Read the model definition and answer for the solid it produces. Units are mm, in the model's axes. A direction names the side the tool comes from. Round coordinates to 2 decimals unless told otherwise and drop trailing zeros. Order: outer loops, then holes, each group sorted by start corner. A loop starts at its lowest first (then second) coordinate and runs counter-clockwise, first axis right, second up. Notation, with made-up numbers: (29, 21) -> (84, 21) arc R32 ccw to (84, 56) -> close; hole circle Ø5 at (-32, 8). An arc over 180 degrees is marked (long way). Use a Markdown table: item, result. Add a question column.
1. Given pin 1 (2.5 mm diameter, centred on x = 3.5, y = 21, fed in from -Z); pin 2 (3 mm diameter, centred on x = -17.5, z = 10.5, fed in from +Y); pin 3 (4 mm diameter, centred on y = 14.5, z = 18.5, fed in from +X), each flat-ended and moving along its own axis, determine where each tip first touches the part or whether it passes through.
2. Section A-A, the plane z = 15.6 is taken. Give the vertices of the cut face in (x, y), then the cut area to 3 significant figures.
3. Section B-B, the plane y = 32 is taken. Give the vertices of the cut face in (x, z).
4. For faces 1 (the face through (-6.6, 5, 15)), 2 (the face through (-14, 33.75, 15)), 3 (the face through (-1, 33.75, 15)), determine the directions among +Z, -Z, +X, -X, +Y, -Y from which every point of the face is accessible in a straight line to the end or side of a thin tool.
5. Section C-C, the plane x = -7.5 is taken. Give the vertices of the cut face in (y, z).
6. Consider L1, parallel to X at y = 35.5, z = 15.25; L2, parallel to X at y = 9, z = 19.5; L3, parallel to Y at x = -3.5, z = 10.75. Determine where each line is inside the solid, lowest interval first. Write a range as [from, to].
7. Section D-D, the plane z = 12.75 is taken. Give the vertices of the cut face in (x, y).
```python
from build123d import *

# Parameters (mm, degrees)
BOX010_W                  = 10
BOX010_H                  = 10
BOX010_DEPTH              = 7
CYLINDER003_R             = 6
CYLINDER003_DEPTH         = 6
CYLINDER003_ROLL_ANGLE    = 90
BOX009_W                  = 26
BOX009_H                  = 23.7
BOX009_DEPTH              = 13
BOX008_W                  = 35
BOX008_H                  = 2
BOX008_DEPTH              = 13
FUSION005_PLACEMENT_ANGLE = -90


with BuildPart() as cube002:
    # Box010 → Box010 (new body)
    with BuildSketch(Plane(origin=(-32, 3.3, 1.3), x_dir=(1, 0, 0), z_dir=(0, 0, 1))):
        with Locations((5, 5)):
            Rectangle(BOX010_W, BOX010_H)
    extrude(amount=BOX010_DEPTH)


with BuildPart() as cylinder003:
    # Cylinder003 → Cylinder003 (new body)
    with BuildSketch(Plane.XY):
        Circle(CYLINDER003_R)
    extrude(amount=CYLINDER003_DEPTH)


with BuildPart() as cylinder003_1:
    # Cylinder003 roll: moved
    add(cylinder003.part.rotate(Axis((0, 0, 0), (1, 0, 0)), CYLINDER003_ROLL_ANGLE))


with BuildPart() as cylinder003_2:
    # Cylinder003 placement: moved
    add(cylinder003_1.part.moved(Location((-31, 14.3, 4.6))))


with BuildPart() as cube001:
    # Box009 → Box009 (new body)
    with BuildSketch(Plane(origin=(-37.75, -13.6, -2), x_dir=(1, 0, 0), z_dir=(0, 0, 1))):
        with Locations((13, 11.85)):
            Rectangle(BOX009_W, BOX009_H)
    extrude(amount=BOX009_DEPTH)


with BuildPart() as simple_servo_rev_eng:
    # Box008 → Box008 (new body)
    with BuildSketch(Plane(origin=(-42, 1.5, -2), x_dir=(1, 0, 0), z_dir=(0, 0, 1))):
        with Locations((17.5, 1)):
            Rectangle(BOX008_W, BOX008_H)
    extrude(amount=BOX008_DEPTH)

    # Fusion005: union Cube002, Cylinder003, Cube001
    add(cube002.part)
    add(cylinder003_2.part)
    add(cube001.part)


with BuildPart() as simple_servo_rev_eng_1:
    # Fusion005 placement: moved
    add(simple_servo_rev_eng.part.moved(Location((-8.1, -4, 11))).rotate(Axis((-8.1, -4, 11), (0, 0, 1)), FUSION005_PLACEMENT_ANGLE))


solid = simple_servo_rev_eng_1.part
```
Verdict:
| question | item | result |
|---|---|---|
| 1 | pin 1 | stops at z = 11.93 |
| 1 | pin 2 | stops at y = 33.75 |
| 1 | pin 3 | stops at x = 2 |
| 2 | outline | (-21.7, 7.75) -> (-6.6, 7.75) -> (-6.6, 3) -> (-4.6, 3) -> (-4.6, 7.75) -> (2, 7.75) -> (2, 18) -> (5.2, 18) -> (5.2, 21) -> (6.2, 21) -> (6.2, 33) -> (2, 33) -> (2, 33.75) -> (-4.6, 33.75) -> (-4.6, 38) -> (-6.6, 38) -> (-6.6, 33.75) -> (-21.7, 33.75) -> close |
| 2 | area | 694 mm2 |
| 3 | outline | (-21.7, 9) -> (2, 9) -> (2, 12.28) -> (6.2, 12.28) -> (6.2, 18.92) -> (2, 18.92) -> (2, 22) -> (-21.7, 22) -> close |
| 4 | face 1 | +Z, -Z, -X, -Y |
| 4 | face 2 | +Z, -Z, -X, +Y |
| 4 | face 3 | +Z, -Z, +X, +Y |
| 5 | outline | (7.75, 9) -> (33.75, 9) -> (33.75, 22) -> (7.75, 22) -> close |
| 6 | L1 | x = [-6.6, -4.6] |
| 6 | L2 | x = [-21.7, 2] |
| 6 | L3 | y = [7.75, 33.75] |
| 7 | outline | (-21.7, 7.75) -> (-6.6, 7.75) -> (-6.6, 3) -> (-4.6, 3) -> (-4.6, 7.75) -> (2, 7.75) -> (2, 18) -> (5.2, 18) -> (5.2, 21.72) -> (6.2, 21.72) -> (6.2, 32.28) -> (2, 32.28) -> (2, 33.75) -> (-4.6, 33.75) -> (-4.6, 38) -> (-6.6, 38) -> (-6.6, 33.75) -> (-21.7, 33.75) -> close |
